For this review, take the finished solid that the model builds, in its own axes (mm). Face numbers are marked on the shaded views. A direction names the side the tool comes from. Round coordinates to 2 decimals unless told otherwise and drop trailing zeros. Loops run counter-clockwise (first coordinate to the right, second up) from the corner with the lowest first, then second, coordinate; pieces in that order, holes last.
1) Wall thickness on L1, parallel to X at y = 10, z = -3.5; L2, parallel to Z at x = 10.5, y = 33; L3, parallel to Z at x = 11, y = 16: over which ranges is each line inside the solid? List them lowest first.
2) Insertion check: pin 1 (8 mm diameter, centred on x = 13.5, y = 21.5, fed in from -Z); pin 2 (1 mm diameter, centred on y = 8.5, z = 1.5, fed in from +X); pin 3 (6 mm diameter, centred on x = -9.5, y = 17, fed in from +Z). Each pin has a flat end and moves straight along its axis. Give the tip position at first contact, or say it passes through.
3) Take a section at A-A (y = 21.5). State the section outline as (x, z) points, then the cut area to 3 significant figures.
4) Tool access review of the marked faces 1 and 2: name each direction out of +Z, -Z, +X, -X, +Y, -Y from which nothing blocks a thin tool from reaching the whole face with its end or side.
5) Take a section at B-B (z = 0). State the section outline as (x, y) points, then the cut area to 3 significant figures.
6) Mouldability with a two-part tool opening along Z and no side actions: class the marked faces 3 and 4 as pulls with the +Z half, pulls with the -Z half, needs draft (parallel to the pull), parting line crosses it, or undercut.
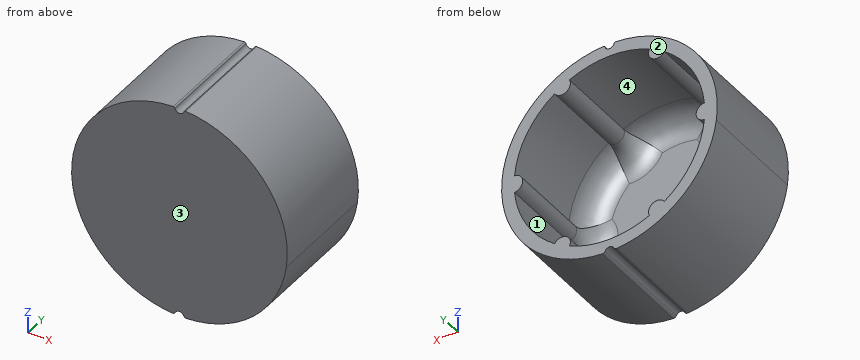
```python
from build123d import *

# Parameters (mm, degrees)
BOSS_EXTRUDE1_DEPTH = 35
CUT_EXTRUDE2_DEPTH  = 36
BOSS_EXTRUDE2_DEPTH = 0.4
FILLET1_R           = 8


with BuildPart() as part:
    # Sketch1 → Boss-Extrude1 (new body)
    with BuildSketch(Plane(origin=(0, 0, 0), x_dir=(1, 0, 0), z_dir=(0, 1, 0))):
        with BuildLine():
            ThreePointArc((1.451818925, -34.068556857), (1.641248992, -34.346908706), (1.964225605, -34.442038138))
            ThreePointArc((1.964225605, -34.442038138), (26.591847487, -21.978073076), (34.198225299, 4.555174015))
            ThreePointArc((34.198225299, 4.555174015), (23.590291339, 25.176355888), (2.324135821, 34.423627607))
            ThreePointArc((2.324135821, 34.423627607), (1.751838249, 34.289058819), (1.354061739, 33.856153382))
            ThreePointArc((1.354061739, 33.856153382), (0, 33.001534515), (-1.354061739, 33.856153382))
            ThreePointArc((-1.354061739, 33.856153382), (-1.751838249, 34.289058819), (-2.324135821, 34.423627607))
            ThreePointArc((-2.324135821, 34.423627607), (-23.590291339, 25.176355888), (-34.198225299, 4.555174015))
            ThreePointArc((-34.198225299, 4.555174015), (-26.591847487, -21.978073076), (-1.964225605, -34.442038138))
            ThreePointArc((-1.964225605, -34.442038138), (-1.641248992, -34.346908706), (-1.451818925, -34.068556857))
            ThreePointArc((-1.451818925, -34.068556857), (0, -32.945679925), (1.451818925, -34.068556857))
        make_face()
        with BuildLine():
            Line((-2.417, 3.787737139), (0, 3.787737139))
            Line((0, 3.787737139), (2.417, 3.787737139))
            ThreePointArc((2.417, 3.787737139), (0, -4.489512172), (-2.417, 3.787737139))
        make_face(mode=Mode.SUBTRACT)
    extrude(amount=BOSS_EXTRUDE1_DEPTH)

    # Sketch2 → Cut-Extrude2 (cut, through all)
    with BuildSketch(Plane(origin=(0, 0, 0), x_dir=(1, 0, 0), z_dir=(0, 1, 0))):
        with BuildLine():
            ThreePointArc((-17.567160793, 24.932806936), (-26.413774815, 15.25), (-30.37602459, 2.747204051))
            ThreePointArc((-30.37602459, 2.747204051), (-27.75, 0), (-30.37602459, -2.747204051))
            ThreePointArc((-30.37602459, -2.747204051), (-26.413774815, -15.25), (-17.567160793, -24.932806936))
            ThreePointArc((-17.567160793, -24.932806936), (-13.875, -24.032204955), (-12.808863798, -27.680010987))
            ThreePointArc((-12.808863798, -27.680010987), (0, -30.5), (12.808863798, -27.680010987))
            ThreePointArc((12.808863798, -27.680010987), (13.875, -24.032204955), (17.567160793, -24.932806936))
            ThreePointArc((17.567160793, -24.932806936), (26.413774815, -15.25), (30.37602459, -2.747204051))
            ThreePointArc((30.37602459, -2.747204051), (27.75, 0), (30.37602459, 2.747204051))
            ThreePointArc((30.37602459, 2.747204051), (26.413774815, 15.25), (17.567160793, 24.932806936))
            ThreePointArc((17.567160793, 24.932806936), (13.875, 24.032204955), (12.808863798, 27.680010987))
            ThreePointArc((12.808863798, 27.680010987), (0, 30.5), (-12.808863798, 27.680010987))
            ThreePointArc((-12.808863798, 27.680010987), (-13.875, 24.032204955), (-17.567160793, 24.932806936))
        make_face()
    extrude(amount=CUT_EXTRUDE2_DEPTH, mode=Mode.SUBTRACT)

    # Sketch2<2> → Boss-Extrude2 (add)
    with BuildSketch(Plane(origin=(0, 0, 0), x_dir=(1, 0, 0), z_dir=(0, 1, 0))):
        with BuildLine():
            ThreePointArc((-17.567160793, 24.932806936), (-26.413774815, 15.25), (-30.37602459, 2.747204051))
            ThreePointArc((-30.37602459, 2.747204051), (-27.75, 0), (-30.37602459, -2.747204051))
            ThreePointArc((-30.37602459, -2.747204051), (-26.413774815, -15.25), (-17.567160793, -24.932806936))
            ThreePointArc((-17.567160793, -24.932806936), (-13.875, -24.032204955), (-12.808863798, -27.680010987))
            ThreePointArc((-12.808863798, -27.680010987), (0, -30.5), (12.808863798, -27.680010987))
            ThreePointArc((12.808863798, -27.680010987), (13.875, -24.032204955), (17.567160793, -24.932806936))
            ThreePointArc((17.567160793, -24.932806936), (26.413774815, -15.25), (30.37602459, -2.747204051))
            ThreePointArc((30.37602459, -2.747204051), (27.75, 0), (30.37602459, 2.747204051))
            ThreePointArc((30.37602459, 2.747204051), (26.413774815, 15.25), (17.567160793, 24.932806936))
            ThreePointArc((17.567160793, 24.932806936), (13.875, 24.032204955), (12.808863798, 27.680010987))
            ThreePointArc((12.808863798, 27.680010987), (0, 30.5), (-12.808863798, 27.680010987))
            ThreePointArc((-12.808863798, 27.680010987), (-13.875, 24.032204955), (-17.567160793, 24.932806936))
        make_face()
    extrude(amount=BOSS_EXTRUDE2_DEPTH)

    # Fillet1
    fillet1_edges = [part.edges().sort_by_distance(p)[0] for p in [
        (26.413774815, 0.4, 15.25),
        (27.75, 0.4, 0),
        (26.413774815, 0.4, -15.25),
        (13.875, 0.4, -24.032204955),
        (0, 0.4, -30.5),
        (-13.875, 0.4, -24.032204955),
        (-26.413774815, 0.4, -15.25),
        (-27.75, 0.4, 0),
        (-26.413774815, 0.4, 15.25),
        (-13.875, 0.4, 24.032204955),
        (0, 0.4, 30.5),
        (13.875, 0.4, 24.032204955),
    ]]
    fillet(fillet1_edges, radius=FILLET1_R)


solid = part.part
```
Response:
1. L1: x = -34.32 to -30.3, 30.3 to 34.32
1. L2: z = -32.87 to -28.64, 28.64 to 32.86
1. L3: z = -32.7 to -28.45, 28.45 to 32.7
2. pin 1: stops at z = -33.17
2. pin 2: stops at x = 34.49
2. pin 3: stops at z = 33.88
3. outline: (-2.32, -34.42) arc R1 ccw to (-1.35, -33.86) arc R1.5 cw to (1.35, -33.86) arc R1 ccw to (2.32, -34.42) arc R34.5 ccw to (1.96, 34.44) arc R0.5 ccw to (1.45, 34.07) arc R1.5 cw to (-1.45, 34.07) arc R0.5 ccw to (-1.96, 34.44) arc R34.5 ccw to start; hole (-30.38, -2.75) arc R30.5 ccw to (-17.57, -24.93) arc R2.75 cw to (-12.81, -27.68) arc R30.5 ccw to (12.81, -27.68) arc R2.75 cw to (17.57, -24.93) arc R30.5 ccw to (30.38, -2.75) arc R2.75 cw to (30.38, 2.75) arc R30.5 ccw to (17.57, 24.93) arc R2.75 cw to (12.81, 27.68) arc R30.5 ccw to (-12.81, 27.68) arc R2.75 cw to (-17.57, 24.93) arc R30.5 ccw to (-30.38, 2.75) arc R2.75 cw to start
3. area: 879 mm2
4. face 1: +Y
4. face 2: +Z, -Z, +X, -X, +Y
5. outline: (-34.5, 0) - (34.5, 0) - (34.5, 35) - (27.75, 35) - (27.75, 8.4) arc R8 cw to (19.75, 0.4) - (-19.75, 0.4) arc R8 cw to (-27.75, 8.4) - (-27.75, 35) - (-34.5, 35) - close
5. area: 522 mm2
6. face 3: needs draft
6. face 4: undercut
